```python
from build123d import *

# Parameters (mm, degrees)
BOX039_W                    = 10.75
BOX039_H                    = 10
BOX039_DEPTH                = 4
BOX038_W                    = 4
BOX038_H                    = 10
BOX038_DEPTH                = 14
FUSION038_ROLL_ANGLE        = 90
FUSION038_PLACEMENT_ANGLE   = 90
PRISM001_DEPTH              = 10
PRISM001_ROLL_ANGLE         = 90.000052
PRISM001_PITCH_ANGLE        = 59.999967
PRISM001_PLACEMENT_ANGLE    = 90.000052
CYLINDER040_R               = 1.5
CYLINDER040_DEPTH           = 28
CYLINDER040_ROLL_ANGLE      = 90.000052
CYLINDER040_PITCH_ANGLE     = 59.999967
CYLINDER040_PLACEMENT_ANGLE = 90.000052
CYLINDER039_R               = 1.5
CYLINDER039_DEPTH           = 28
CYLINDER039_PITCH_ANGLE     = 90
PRISM002_DEPTH              = 10
PRISM002_ROLL_ANGLE         = 90.000052
PRISM002_PITCH_ANGLE        = 59.999967
PRISM002_PLACEMENT_ANGLE    = 90.000052
PAD019_DEPTH                = 34
FILLET031_R                 = 7
FILLET032_R                 = 3
SKETCH021_W                 = 40
SKETCH021_H                 = 16
SKETCH021_R                 = 1.4
PAD018_DEPTH                = 3
FILLET033_R                 = 0.5


with BuildPart() as cube039:
    # Box039 → Box039 (new body)
    with BuildSketch(Plane(origin=(-5, -3, -10.5), x_dir=(1, 0, 0), z_dir=(0, 0, 1))):
        with Locations((5.375, 5)):
            Rectangle(BOX039_W, BOX039_H)
    extrude(amount=BOX039_DEPTH)


with BuildPart() as fusion038:
    # Box038 → Box038 (new body)
    with BuildSketch(Plane(origin=(-2.5, -3, 0), x_dir=(1, 0, 0), z_dir=(0, 0, 1))):
        with Locations((2, 5)):
            Rectangle(BOX038_W, BOX038_H)
    extrude(amount=BOX038_DEPTH)

    # Fusion038: union Cube039
    add(cube039.part)


with BuildPart() as fusion038_1:
    # Fusion038 roll: moved
    add(fusion038.part.rotate(Axis((0, 0, 0), (1, 0, 0)), FUSION038_ROLL_ANGLE))


with BuildPart() as fusion038_2:
    # Fusion038 placement: moved
    add(fusion038_1.part.moved(Location((-7, 0, 5))).rotate(Axis((-7, 0, 5), (0, 0, 1)), FUSION038_PLACEMENT_ANGLE))


with BuildPart() as prism001:
    # Prism001 → Prism001 (new body)
    with BuildSketch(Plane.XY):
        Polygon((3.2, 0), (1.6, 2.771281), (-1.6, 2.771281), (-3.2, 0), (-1.6, -2.771281), (1.6, -2.771281), align=None)
    extrude(amount=PRISM001_DEPTH)


with BuildPart() as prism001_1:
    # Prism001 roll: moved
    add(prism001.part.rotate(Axis((0, 0, 0), (1, 0, 0)), PRISM001_ROLL_ANGLE))


with BuildPart() as prism001_2:
    # Prism001 pitch: moved
    add(prism001_1.part.rotate(Axis((0, 0, 0), (0, 1, 0)), PRISM001_PITCH_ANGLE))


with BuildPart() as prism001_3:
    # Prism001 placement: moved
    add(prism001_2.part.moved(Location((-16, -19, -12))).rotate(Axis((-16, -19, -12), (0, 0, 1)), PRISM001_PLACEMENT_ANGLE))


with BuildPart() as cylinder040:
    # Cylinder040 → Cylinder040 (new body)
    with BuildSketch(Plane.XY):
        Circle(CYLINDER040_R)
    extrude(amount=CYLINDER040_DEPTH)


with BuildPart() as cylinder040_1:
    # Cylinder040 roll: moved
    add(cylinder040.part.rotate(Axis((0, 0, 0), (1, 0, 0)), CYLINDER040_ROLL_ANGLE))


with BuildPart() as cylinder040_2:
    # Cylinder040 pitch: moved
    add(cylinder040_1.part.rotate(Axis((0, 0, 0), (0, 1, 0)), CYLINDER040_PITCH_ANGLE))


with BuildPart() as cylinder040_3:
    # Cylinder040 placement: moved
    add(cylinder040_2.part.moved(Location((-16, -19, -12))).rotate(Axis((-16, -19, -12), (0, 0, 1)), CYLINDER040_PLACEMENT_ANGLE))


with BuildPart() as cylinder039:
    # Cylinder039 → Cylinder039 (new body)
    with BuildSketch(Plane.XY):
        Circle(CYLINDER039_R)
    extrude(amount=CYLINDER039_DEPTH)


with BuildPart() as cylinder039_1:
    # Cylinder039 pitch: moved
    add(cylinder039.part.rotate(Axis((0, 0, 0), (0, 1, 0)), CYLINDER039_PITCH_ANGLE))


with BuildPart() as cylinder039_2:
    # Cylinder039 placement: moved
    add(cylinder039_1.part.moved(Location((-12, 1, -12))))


with BuildPart() as fusion037:
    # Prism002 → Prism002 (new body)
    with BuildSketch(Plane.XY):
        Polygon((3.2, 0), (1.6, 2.771281), (-1.6, 2.771281), (-3.2, 0), (-1.6, -2.771281), (1.6, -2.771281), align=None)
    extrude(amount=PRISM002_DEPTH)


with BuildPart() as fusion037_1:
    # Prism002 roll: moved
    add(fusion037.part.rotate(Axis((0, 0, 0), (1, 0, 0)), PRISM002_ROLL_ANGLE))


with BuildPart() as fusion037_2:
    # Prism002 pitch: moved
    add(fusion037_1.part.rotate(Axis((0, 0, 0), (0, 1, 0)), PRISM002_PITCH_ANGLE))


with BuildPart() as fusion037_3:
    # Prism002 placement: moved
    add(fusion037_2.part.moved(Location((-16, 1, -12))).rotate(Axis((-16, 1, -12), (0, 0, 1)), PRISM002_PLACEMENT_ANGLE))

    # Fusion037: union Prism001, Cylinder040, Cylinder039
    add(prism001_3.part)
    add(cylinder040_3.part)
    add(cylinder039_2.part)


with BuildPart() as fillet032:
    # Sketch022 → Pad019 (new body)
    with BuildSketch(Plane.XZ.offset(-8)):
        with BuildLine():
            Line((-8, -16), (-8, 3))
            Line((-8, 3), (8, 3))
            Line((8, 3), (8, -16))
            Line((8, -16), (4.5, -16))
            Line((4.5, -16), (4.5, -7.179449))
            ThreePointArc((4.5, -7.179449), (0, 0), (-4.5, -7.179449))
            Line((-4.5, -7.179449), (-4.5, -16))
            Line((-4.5, -16), (-8, -16))
        make_face()
    extrude(amount=PAD019_DEPTH)

    # Fillet031
    fillet031_edges = [fillet032.edges().sort_by_distance(p)[0] for p in [
        (-8, -9, 3),
        (8, -9, 3),
    ]]
    fillet(fillet031_edges, radius=FILLET031_R)

    # Fillet032
    fillet032_edges = [fillet032.edges().sort_by_distance(p)[0] for p in [
        (-6.25, 8, -16),
        (6.25, 8, -16),
        (-6.25, -26, -16),
        (6.25, -26, -16),
    ]]
    fillet(fillet032_edges, radius=FILLET032_R)


with BuildPart() as cut042:
    # Sketch021 → Pad018 (new body)
    with BuildSketch(Plane.XY):
        with Locations((-6.8, 0)):
            Rectangle(SKETCH021_W, SKETCH021_H)
        with Locations((-9.5, 5)):
            Circle(SKETCH021_R, mode=Mode.SUBTRACT)
        with Locations((9.5, 5)):
            Circle(SKETCH021_R, mode=Mode.SUBTRACT)
    extrude(amount=PAD018_DEPTH)

    # Fusion036: union Fillet032
    add(fillet032.part)

    # Cut041: cut Fusion037
    add(fusion037_3.part, mode=Mode.SUBTRACT)

    # Fillet033
    fillet033_edges = [cut042.edges().sort_by_distance(p)[0] for p in [
        (-26.8, -8, 1.5),
        (-26.8, 8, 1.5),
        (13.2, 8, 1.5),
        (-6.744563, 0, 0),
        (13.2, -8, 1.5),
        (6.744563, 0, 0),
    ]]
    fillet(fillet033_edges, radius=FILLET033_R)

    # Cut042: cut Fusion038
    add(fusion038_2.part, mode=Mode.SUBTRACT)


solid = cut042.part
```
Work out the finished part from the listing and answer in its coordinate system (mm). A direction names the side the tool comes from. Give positions to 0.01 mm unless a question says otherwise; leave off trailing zeros. Write each loop counter-clockwise with the first axis right and the second up, starting at its lowest first coordinate (ties: lowest second). Pieces come first, ordered by that corner, then holes.
(1) The mould has two halves that part along Y. Classify faces 5 (the cylindrical face through (-10.9, 5.06, 1.48)), 6 (the flat face through (-17, -8, 2)), 7 (the flat face through (-7.014, -1.389, -10.595)), 8 (the flat face through (13.2, 0, 1)): pulls with the +Y half, pulls with the -Y half, needs draft (parallel to the pull), parting line crosses it, or undercut.
Final values:
face 5: undercut
face 6: pulls with the -Y half
face 7: undercut
face 8: needs draft
(2) The part is cut by section C-C on y = -9.5. Write down the section's boundary in (x, z).
Final values:
outline: (-8, -16) - (-4.5, -16) - (-4.5, -7.18) arc R5 cw (long way) to (4.5, -7.18) - (4.5, -16) - (8, -16) - (8, -4) arc R7 ccw to (1, 3) - (-1, 3) arc R7 ccw to (-8, -4) - close
(3) Flat-ended cylindrical pins translate along their axes: pin 1 Ø4 at (y, z) = (1, -12) entering from -X; pin 2 Ø1 at (x, y) = (2, -14.5) entering from +Z; pin 3 Ø7 at (y, z) = (-1.5, -10.5) entering from -X. Find the tip coordinate at first contact, or state that the pin passes through.
Final values:
pin 1: stops at x = -6
pin 2: stops at z = 2.98
pin 3: stops at x = -8
(4) Straight lines are drawn through the part: line 1 (Y direction, x = 6.9, z = -12); line 2 (Y direction, x = -9.5, z = 1.25); line 3 (X direction, y = 4.5, z = -8.5). For each, find the intervals that lie inside material, in ascending order.
Final values:
line 1: y = -26 to -20.5, -17.5 to -0.5, 2.5 to 8
line 2: y = -8 to 3.6, 6.4 to 8
line 3: x = -8 to -4.5, 4.5 to 8
(5) The part is cut by section D-D on x = 0. Write down the section's boundary in (y, z), plus the area to 3 significant figures.
Final values:
outline: (-26, 0) - (8, 0) - (8, 3) - (1.5, 3) - (1.5, 2) - (-2.5, 2) - (-2.5, 3) - (-26, 3) - close
area: 98.0 mm2
(6) The part is cut by section A-A on x = -9.5. Write down the section's boundary in (y, z), plus the area to 3 significant figures.
Final values:
outline: (-8, 0) - (3.6, 0) - (3.6, 3) - (-8, 3) - close; (6.4, 0) - (8, 0) - (8, 3) - (6.4, 3) - close
area: 39.6 mm2
(7) The part is cut by section B-B on z = -5. Write down the section's boundary in (x, y).
Final values:
outline: (-8, -26) - (-5, -26) - (-5, 8) - (-8, 8) - close; (5, -26) - (8, -26) - (8, 8) - (5, 8) - close
(8) Which of the six approach directions +Z, -Z, +X, -X, +Y, -Y give full straight-line access (tool end or side, diameter ignored) to faces 1 (the flat face through (8, -9, -10)), 2 (the flat face through (-15.5, -5, 2.5)), 3 (the flat face through (-8, -9, -10)), 4 (the flat face through (4.5, -9, -12))?
Final values:
face 1: -Z, +X, +Y, -Y
face 2: +Z
face 3: -Z, -X, +Y, -Y
face 4: -Z, +Y, -Y
